from build123d import *

# Parameters (mm, degrees)
SKETCH1_W           = 42.5
SKETCH1_H           = 27
BOSS_EXTRUDE1_DEPTH = 6
SKETCH2_W           = 40.5
SKETCH2_H           = 25
CUT_EXTRUDE1_DEPTH  = 4
SKETCH3_W           = 6.4
SKETCH3_H           = 6.4
CUT_EXTRUDE2_DEPTH  = 5
CUT_EXTRUDE3_REACH  = 44.5
SKETCH4_R           = 1.75
SKETCH5_W           = 8.5
SKETCH5_H           = 25
CUT_EXTRUDE4_DEPTH  = 1
SKETCH6_W           = 8
SKETCH6_H           = 4
CUT_EXTRUDE5_DEPTH  = 1
SKETCH7_W           = 4.5
SKETCH7_H           = 3
CUT_EXTRUDE6_DEPTH  = 1
FILLET1_R           = 1.5
FILLET2_R           = 2.5
SKETCH8_W           = 6.4
SKETCH8_H           = 8.4
CUT_EXTRUDE7_DEPTH  = 1


with BuildPart() as part:
    # Sketch1 → Boss-Extrude1 (new body)
    with BuildSketch(Plane(origin=(0, 0, 0), x_dir=(1, 0, 0), z_dir=(0, 1, 0))):
        Rectangle(SKETCH1_W, SKETCH1_H)
    extrude(amount=BOSS_EXTRUDE1_DEPTH)

    # Sketch2 → Cut-Extrude1 (cut)
    with BuildSketch(Plane(origin=(0, 6, 0), x_dir=(1, 0, 0), z_dir=(0, 1, 0))):
        Rectangle(SKETCH2_W, SKETCH2_H)
    extrude(amount=-CUT_EXTRUDE1_DEPTH, mode=Mode.SUBTRACT)

    # Sketch3 → Cut-Extrude2 (cut)
    with BuildSketch(Plane(origin=(0, 6, 0), x_dir=(1, 0, 0), z_dir=(0, 1, 0))):
        with Locations((18.05, 0)):
            Rectangle(SKETCH3_W, SKETCH3_H)
    extrude(amount=-CUT_EXTRUDE2_DEPTH, mode=Mode.SUBTRACT)

    # Sketch4 → Cut-Extrude3 (cut, up to next)
    with BuildSketch(Plane.ZY.offset(21.25), mode=Mode.PRIVATE) as cut_extrude3_sk1:
        with Locations((0, 6)):
            Circle(SKETCH4_R)
    cut_extrude3_tool1 = extrude(cut_extrude3_sk1.sketch, amount=-CUT_EXTRUDE3_REACH, mode=Mode.PRIVATE) & part.part
    add(cut_extrude3_tool1.solids().sort_by_distance((-21.25, 6, 0))[0], mode=Mode.SUBTRACT)

    # Sketch5 → Cut-Extrude4 (cut)
    with BuildSketch(Plane(origin=(0, 2, 0), x_dir=(1, 0, 0), z_dir=(0, 1, 0))):
        with Locations((-5, 0)):
            Rectangle(SKETCH5_W, SKETCH5_H)
    extrude(amount=-CUT_EXTRUDE4_DEPTH, mode=Mode.SUBTRACT)

    # Sketch6 → Cut-Extrude5 (cut)
    with BuildSketch(Plane(origin=(0, 2, 0), x_dir=(1, 0, 0), z_dir=(0, 1, 0))):
        with Locations((-16.25, 0)):
            Rectangle(SKETCH6_W, SKETCH6_H)
    extrude(amount=-CUT_EXTRUDE5_DEPTH, mode=Mode.SUBTRACT)

    # Sketch7 → Cut-Extrude6 (cut)
    with BuildSketch(Plane(origin=(0, 2, 0), x_dir=(1, 0, 0), z_dir=(0, 1, 0))):
        with Locations((-14, -5.5)):
            Rectangle(SKETCH7_W, SKETCH7_H)
    extrude(amount=-CUT_EXTRUDE6_DEPTH, mode=Mode.SUBTRACT)

    # Fillet1
    fillet1_edges = [part.edges().sort_by_distance(p)[0] for p in [
        (20.25, 4, -12.5),
        (20.25, 4, 12.5),
        (-20.25, 4, 12.5),
        (-20.25, 4, -12.5),
    ]]
    fillet(fillet1_edges, radius=FILLET1_R)

    # Fillet2
    fillet2_edges = [part.edges().sort_by_distance(p)[0] for p in [
        (21.25, 3, 13.5),
        (-21.25, 3, 13.5),
        (-21.25, 3, -13.5),
        (21.25, 3, -13.5),
    ]]
    fillet(fillet2_edges, radius=FILLET2_R)

    # Sketch8 → Cut-Extrude7 (cut)
    with BuildSketch(Plane(origin=(0, 2, 0), x_dir=(1, 0, 0), z_dir=(0, 1, 0))):
        with Locations((17.05, 0)):
            Rectangle(SKETCH8_W, SKETCH8_H)
    extrude(amount=-CUT_EXTRUDE7_DEPTH, mode=Mode.SUBTRACT)


solid = part.part
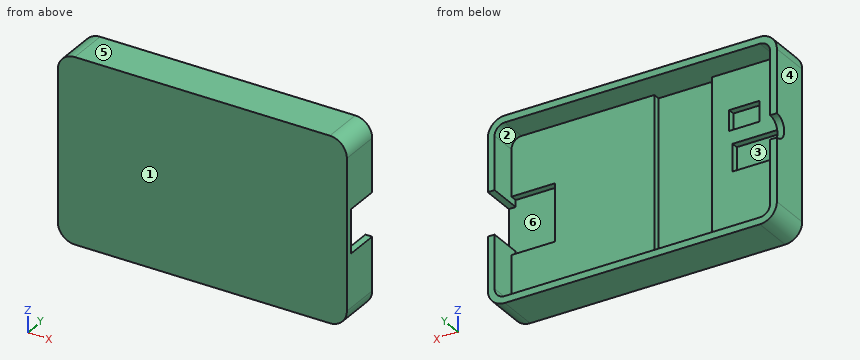
Geometry: final body of the model. Coordinates: model frame, mm. Face numbers are marked on the shaded views. A direction names the side the tool comes from. Give positions to 0.01 mm unless a question says otherwise; leave off trailing zeros. Write each loop counter-clockwise with the first axis right and the second up, starting at its lowest first coordinate (ties: lowest second). Pieces come first, ordered by that corner, then holes.
(1) Cut plane B-B, the plane x = -5. Return loops of the section in (y, z), then the cut area to 3 significant figures.
(2) Access query for the marked faces 1 and 2. Directions: +Z, -Z, +X, -X, +Y, -Y. A direction counts if a zero-diameter tool reaches every point of the face in a straight line with its end or side. Return the directions, or none.
(3) Cut plane A-A, the plane z = 10.5. Return loops of the section in (x, y), then the cut area to 3 significant figures.
(4) Cut plane D-D, the plane y = 2.75. Return loops of the section in (x, z).
(5) First-contact query: P1, Ø3.5, axis at x = 16.5, z = 0.5, coming from the +Y side; P2, Ø10.5, axis at x = 6.5, z = -1, coming from the +Y side; P3, Ø3, axis at y = 4.5, z = 0.5, coming from the +X side. Flat tips, straight axial feed; report the tip coordinate or a pass-through.
(6) Cut plane C-C, the plane y = 5.2. Return loops of the section in (x, z), then the cut area to 3 significant figures.
(7) Mould query, pull axis X, two halves, no side actions, for the marked faces 3, 4, 5 and 6. Classes: released by +X, released by -X, zero draft, split by the parting line, or undercut.
(8) Ray query, line 1 (X direction, y = 1.95, z = 5.5); line 2 (X direction, y = 1.65, z = 2.25); line 3 (X direction, y = 1.85, z = -4.25). Return the intervals inside material, ascending.
Values follow:
1. outline: (0, -13.5) - (6, -13.5) - (6, -12.5) - (1, -12.5) - (1, 12.5) - (6, 12.5) - (6, 13.5) - (0, 13.5) - close
1. area: 37.0 mm2
2. face 1: +Z, -Z, +X, -X, -Y
2. face 2: +Y
3. outline: (-21.25, 0) - (21.25, 0) - (21.25, 6) - (20.25, 6) - (20.25, 2) - (-0.75, 2) - (-0.75, 1) - (-9.25, 1) - (-9.25, 2) - (-20.25, 2) - (-20.25, 6) - (-21.25, 6) - close
3. area: 84.5 mm2
4. outline: (-21.25, -11) arc R2.5 ccw to (-18.75, -13.5) - (18.75, -13.5) arc R2.5 ccw to (21.25, -11) - (21.25, -3.2) - (20.25, -3.2) - (20.25, -11) arc R1.5 cw to (18.75, -12.5) - (-18.75, -12.5) arc R1.5 cw to (-20.25, -11) - (-20.25, 11) arc R1.5 cw to (-18.75, 12.5) - (18.75, 12.5) arc R1.5 cw to (20.25, 11) - (20.25, 3.2) - (21.25, 3.2) - (21.25, 11) arc R2.5 ccw to (18.75, 13.5) - (-18.75, 13.5) arc R2.5 ccw to (-21.25, 11) - close
5. P1: stops at y = 1
5. P2: stops at y = 2
5. P3: stops at x = -20.25
6. outline: (-21.25, -11) arc R2.5 ccw to (-18.75, -13.5) - (18.75, -13.5) arc R2.5 ccw to (21.25, -11) - (21.25, -3.2) - (20.25, -3.2) - (20.25, -11) arc R1.5 cw to (18.75, -12.5) - (-18.75, -12.5) arc R1.5 cw to (-20.25, -11) - (-20.25, -1.56) - (-21.25, -1.56) - close; (-21.25, 1.56) - (-20.25, 1.56) - (-20.25, 11) arc R1.5 cw to (-18.75, 12.5) - (18.75, 12.5) arc R1.5 cw to (20.25, 11) - (20.25, 3.2) - (21.25, 3.2) - (21.25, 11) arc R2.5 ccw to (18.75, 13.5) - (-18.75, 13.5) arc R2.5 ccw to (-21.25, 11) - close
6. area: 122 mm2
7. face 3: undercut
7. face 4: released by -X
7. face 5: zero draft
7. face 6: undercut
8. line 1: x = -21.25 to -16.25, -11.75 to -9.25, -0.75 to 21.25
8. line 2: x = -21.25 to -9.25, -0.75 to 13.85
8. line 3: x = -21.25 to -9.25, -0.75 to 21.25
